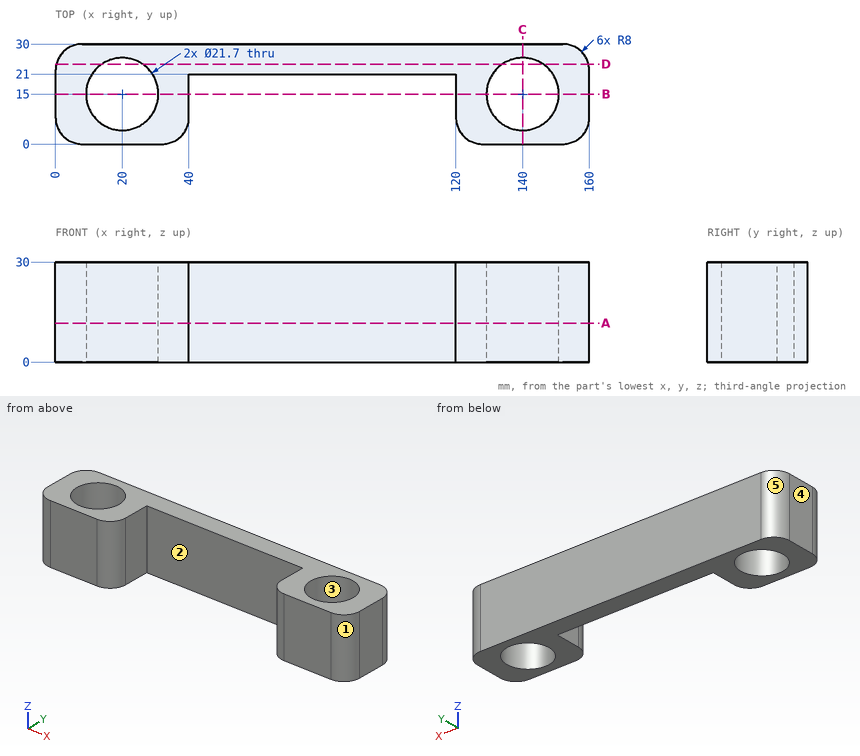
The drawing under review shows one solid part. Ordinate dimensions are in mm from its lowest x, y, z. A direction names the side the tool comes from. Give positions to 0.01 mm unless a question says otherwise; leave off trailing zeros. Write each loop counter-clockwise with the first axis right and the second up, starting at its lowest first coordinate (ties: lowest second). Pieces come first, ordered by that corner, then holes. Notation, with made-up numbers: (9, 38) -> (56, 38) arc R17 cw to (56, 47) -> close; hole circle Ø4 at (73, 89.25). An arc over 180 degrees is marked (long way). Use CSV: the item, a comma, the result in double quotes.
Q1. Take a section at B-B, the plane y = 15. Write out the cut boundary in (x, z).
Conclusion:
outline,"(0, 0) -> (9.15, 0) -> (9.15, 30) -> (0, 30) -> close; (30.85, 0) -> (40, 0) -> (40, 30) -> (30.85, 30) -> close; (120, 0) -> (129.15, 0) -> (129.15, 30) -> (120, 30) -> close; (150.85, 0) -> (160, 0) -> (160, 30) -> (150.85, 30) -> close"
Q2. Take a section at C-C, the plane x = 140. Write out the cut boundary in (y, z).
Conclusion:
outline,"(0, 0) -> (4.15, 0) -> (4.15, 30) -> (0, 30) -> close; (25.85, 0) -> (30, 0) -> (30, 30) -> (25.85, 30) -> close"
Q3. For P1, Ø4, axis at x = 59.5, z = 14.5, coming from the -Y side, flat-tipped, find the tip position at first contact; note if it passes through.
Conclusion:
P1,"y = 21"
Q4. Take a section at D-D, the plane y = 24. Write out the cut boundary in (x, z), then the cut area to 3 significant figures.
Conclusion:
outline,"(0.25, 0) -> (13.94, 0) -> (13.94, 30) -> (0.25, 30) -> close; (26.06, 0) -> (133.94, 0) -> (133.94, 30) -> (26.06, 30) -> close; (146.06, 0) -> (159.75, 0) -> (159.75, 30) -> (146.06, 30) -> close"
area,"4,060 mm2"
Q5. Mouldability with a two-part tool opening along Y and no side actions: class the marked faces 3, 4 and 5 as pulls with the +Y half, pulls with the -Y half, needs draft (parallel to the pull), parting line crosses it, or undercut.
Conclusion:
face 3,"undercut"
face 4,"needs draft"
face 5,"pulls with the +Y half"
Q6. To check wall thickness, follow probe 1 along Y at (x, z) = (140, 8); probe 2 along X at (y, z) = (16, 26); probe 3 along X at (y, z) = (18.5, 6.5). State the ranges of each line that lie inside material, in increasing order. Write a range as [from, to].
Conclusion:
probe 1,"[0, 4.15], [25.85, 30]"
probe 2,"[0, 9.2], [30.8, 40], [120, 129.2], [150.8, 160]"
probe 3,"[0, 9.73], [30.27, 40], [120, 129.73], [150.27, 160]"
Q7. Tool access review of the marked faces 1 and 2: name each direction out of +Z, -Z, +X, -X, +Y, -Y from which nothing blocks a thin tool from reaching the whole face with its end or side.
Conclusion:
face 1,"+Z, -Z, +X, -Y"
face 2,"+Z, -Z, -Y"
Q8. Take a section at A-A, the plane z = 11.75. Write out the cut boundary in (x, y), then the cut area to 3 significant figures.
Conclusion:
outline,"(0, 8) arc R8 ccw to (8, 0) -> (32, 0) arc R8 ccw to (40, 8) -> (40, 21) -> (120, 21) -> (120, 8) arc R8 ccw to (128, 0) -> (152, 0) arc R8 ccw to (160, 8) -> (160, 22) arc R8 ccw to (152, 30) -> (8, 30) arc R8 ccw to (0, 22) -> close; hole circle Ø21.7 at (20, 15); hole circle Ø21.7 at (140, 15)"
area,"2,300 mm2"
